```python
from build123d import *

# Parameters (mm, degrees)
F0_W          = 5.08
F0_H          = 5.08
F1_DEPTH      = 36.83
F1_DEPTH_BACK = 75.184
F2_W          = 2.54
F2_H          = 109.474
F3_DEPTH      = 23.114
F4_W          = 2.54
F4_H          = 109.474
F5_DEPTH      = 4.5777483376
F5_DEPTH_BACK = 29.972
F6_T1_DEPTH   = 124.714


# Not quite as in the source:
# - a fillet or chamfer that OpenCascade refuses, or shapes differently, is made with other operations: its cross-section is extruded or revolved along the edge and cut away or added


with BuildPart() as f1:
    # F0 (on Top) → F1 (new body, two sides)
    with BuildSketch(Plane.XY) as f1_sk:
        with Locations((-2.0367483376, -3.0882195887)):
            Rectangle(F0_W, F0_H)
    extrude(amount=F1_DEPTH)
    extrude(f1_sk.sketch, amount=-F1_DEPTH_BACK)

    # F2 (on Front) → F3 (cut)
    with BuildSketch(Plane.XZ):
        with Locations((-2.0367483376, -19.177)):
            Rectangle(F2_W, F2_H)
    extrude(amount=F3_DEPTH, mode=Mode.SUBTRACT)

    # F4 (on Right) → F5 (cut, two sides)
    with BuildSketch(Plane.YZ) as f5_sk:
        with Locations((-3.0882195887, -19.177)):
            Rectangle(F4_W, F4_H)
    extrude(amount=-F5_DEPTH, mode=Mode.SUBTRACT)
    extrude(f5_sk.sketch, amount=F5_DEPTH_BACK, mode=Mode.SUBTRACT)

    # F6: fillet of radius 2.54 on 4 edges, made by hand

    # F6_s2 → F6_t1 (cut)
    with BuildSketch(Plane.XY.offset(-81.534)):
        with BuildLine():
            ThreePointArc((0.5032516624, -3.0882195887), (-0.2406971133, -4.8842708129), (-2.0367483376, -5.6282195887))
            Line((-2.0367483376, -5.6282195887), (0.5032516624, -5.6282195887))
            Line((0.5032516624, -5.6282195887), (0.5032516624, -3.0882195887))
        make_face()
        with BuildLine():
            ThreePointArc((-4.5767483376, -3.0882195887), (-3.8327995618, -4.8842708129), (-2.0367483376, -5.6282195887))
            Line((-2.0367483376, -5.6282195887), (-4.5767483376, -5.6282195887))
            Line((-4.5767483376, -5.6282195887), (-4.5767483376, -3.0882195887))
        make_face()
        with BuildLine():
            ThreePointArc((-2.0367483376, -0.5482195887), (-3.8327995618, -1.2921683645), (-4.5767483376, -3.0882195887))
            Line((-4.5767483376, -3.0882195887), (-4.5767483376, -0.5482195887))
            Line((-4.5767483376, -0.5482195887), (-2.0367483376, -0.5482195887))
        make_face()
        with BuildLine():
            ThreePointArc((-2.0367483376, -0.5482195887), (-0.2406971133, -1.2921683645), (0.5032516624, -3.0882195887))
            Line((0.5032516624, -3.0882195887), (0.5032516624, -0.5482195887))
            Line((0.5032516624, -0.5482195887), (-2.0367483376, -0.5482195887))
        make_face()
    extrude(amount=F6_T1_DEPTH, mode=Mode.SUBTRACT)


solid = f1.part
```
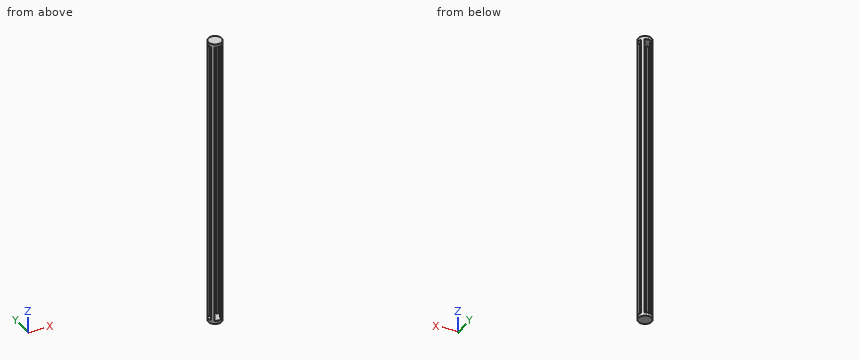
Geometry check sheet. Reference: the model listing, model coordinates, mm. Coordinates: 2 decimals unless noted, no trailing zeros. Order: outer loops, then holes, each group sorted by start corner. A loop starts at its lowest first (then second) coordinate and runs counter-clockwise, first axis right, second up.
Item 1: Scan lines: line 1 along Z through (x, y) = (-1.4, -1.3); line 2 along X through (y, z) = (-1.75, -39); line 3 along X through (y, z) = (-1.5, -48.5). Record each from-to range of solid material in increasing order.
Item 2: Section check A-A (z = -30). Enter the section's corners in (x, y).
Item 3: Depth check by flat-ended pin: pin 1 (1.5 mm diameter, centred on y = -3, z = 9, fed in from -X); pin 2 (0.7 mm diameter, centred on x = -0.5, z = -45, fed in from +Y); pin 3 (0.5 mm diameter, centred on y = -5, z = 5.5, fed in from +X); pin 4 (1.5 mm diameter, centred on y = -1.5, z = 4.5, fed in from -X). Enter the tip coordinate at first touch or a pass-through.
Check sheet entries:
1. line 1: z = -75.18 to -73.91, 35.56 to 36.83
1. line 2: x = -4.2 to -3.31, -0.77 to 0.12
1. line 3: x = -4.02 to -3.31, -0.77 to -0.05
2. outline: (-4.24, -4.36) arc R2.54 ccw to (-3.31, -5.29) - (-3.31, -4.36) - close; (-4.24, -1.82) - (-3.31, -1.82) - (-3.31, -0.89) arc R2.54 ccw to start; (-0.77, -5.29) arc R2.54 ccw to (0.16, -4.36) - (-0.77, -4.36) - close; (-0.77, -1.82) - (0.16, -1.82) arc R2.54 ccw to (-0.77, -0.89) - close
3. pin 1: passes through
3. pin 2: stops at y = -0.89
3. pin 3: stops at x = -0.12
3. pin 4: stops at x = -4.24
